from build123d import *

# Parameters (mm, degrees)
SKETCH1_R           = 7.9375
BOSS_EXTRUDE1_DEPTH = 42
SKETCH4_R           = 19
SKETCH4_R_2         = 2
BOSS_EXTRUDE3_DEPTH = 3.8
BOSS_EXTRUDE5_DEPTH = 19.8272
SKETCH7_R           = 7.9375
BOSS_EXTRUDE6_DEPTH = 24


with BuildPart() as part:
    # Sketch1 → Boss-Extrude1 (new body)
    with BuildSketch(Plane(origin=(0, 0, 0), x_dir=(0, 0, -1), z_dir=(1, 0, 0))):
        Circle(SKETCH1_R)
    extrude(amount=BOSS_EXTRUDE1_DEPTH)

    # Sketch4 → Boss-Extrude3 (add)
    with BuildSketch(Plane.ZY):
        Circle(SKETCH4_R)
        with Locations((-10.5, 10.5)):
            Circle(SKETCH4_R_2, mode=Mode.SUBTRACT)
        with Locations((10.5, 10.5)):
            Circle(SKETCH4_R_2, mode=Mode.SUBTRACT)
        with Locations((10.5, -10.5)):
            Circle(SKETCH4_R_2, mode=Mode.SUBTRACT)
        with Locations((-10.5, -10.5)):
            Circle(SKETCH4_R_2, mode=Mode.SUBTRACT)
    extrude(amount=BOSS_EXTRUDE3_DEPTH)

    # Sketch6 → Boss-Extrude5 (add)
    with BuildSketch(Plane(origin=(42, 0, 0), x_dir=(0, 0, -1), z_dir=(1, 0, 0))):
        with BuildLine():
            Line((-2.3815, 5.188813785), (2.3815, 5.188813785))
            Line((2.3815, 5.188813785), (2.3815, 7.571813785))
            ThreePointArc((2.3815, 7.571813785), (0, -7.9375), (-2.3815, 7.571813785))
            Line((-2.3815, 7.571813785), (-2.3815, 5.188813785))
        make_face()
    extrude(amount=BOSS_EXTRUDE5_DEPTH)

    # Sketch7 → Boss-Extrude6 (add)
    with BuildSketch(Plane(origin=(61.8272, 0, 0), x_dir=(0, 0, -1), z_dir=(1, 0, 0))):
        Circle(SKETCH7_R)
    extrude(amount=BOSS_EXTRUDE6_DEPTH)


solid = part.part
Part model, mm, in its own coordinate system. A direction names the side the tool comes from. Round coordinates to 2 decimals unless told otherwise and drop trailing zeros. Write each loop counter-clockwise with the first axis right and the second up, starting at its lowest first coordinate (ties: lowest second). Pieces come first, ordered by that corner, then holes. Notation, with made-up numbers: M 70.5,23 L 90.5,23 A20 cw 90.5,53 Z; hole C 50,56 d8. An arc over 180 degrees is marked long. Return JSON: item names as keys, results as strings. Group by question number.
(1) Pin check, flat tips, straight feed: pin 1 Ø0.7 at (x, y) = (49.5, 6.5) entering from +Z; pin 2 Ø6.5 at (y, z) = (-10.5, 10.5) entering from +X; pin 3 Ø1.2 at (x, y) = (51, 6) entering from -Z; pin 4 Ø3.5 at (y, z) = (10.5, -10.5) entering from +X. Stop position of each tip, or through.
(2) Saw through at B-B on y = 0. Write the cut outline in (x, z), then the cut area to 3 significant figures.
(3) Saw through at A-A on z = -10.5. Write the cut outline in (x, y).
(4) Two-plate mould, pull along X, no slides. Class faces 3 (the face through (0, 0.3, 8.2)), 4 (the face through (42, 7, 0)), 5 (the face through (-1.873, -9.148, 9.026)): +X half, -X half, draft (parallel to the pull), parting line (faces both ways), or undercut.
(5) Saw through at C-C on z = 0. Write the cut outline in (x, y).
(6) Which spindle directions (+Z, -Z, +X, -X, +Y, -Y) get a long thin tool onto all of the face, cutting with end or side? Do faces 1 (the face through (-1.873, -9.148, -11.974)), 2 (the face through (52, 6, 2.382)). Say none if no direction does.
(7) Drill centre lines: probe 1 along Z at (x, y) = (-1, -10); probe 2 along Y at (x, z) = (-2.4, 10.5); probe 3 along X at (y, z) = (-11, -5). Where is each one in solid material? Low to high.
Returned:
{
 "1": {"pin 1": "z = 5.02", "pin 2": "x = 0", "pin 3": "z = -5.82", "pin 4": "through"},
 "2": {"outline": "M -3.8,-19 L 0,-19 L 0,-7.94 L 85.83,-7.94 L 85.83,7.94 L 0,7.94 L 0,19 L -3.8,19 Z", "area": "1,510 mm²"},
 "3": {"outline": "M -3.8,-15.84 L 0,-15.84 L 0,-12.5 L -3.8,-12.5 Z; M -3.8,-8.5 L 0,-8.5 L 0,8.5 L -3.8,8.5 Z; M -3.8,12.5 L 0,12.5 L 0,15.84 L -3.8,15.84 Z"},
 "4": {"face 3": "+X half", "face 4": "undercut", "face 5": "draft"},
 "5": {"outline": "M -3.8,-19 L 0,-19 L 0,-7.94 L 85.83,-7.94 L 85.83,7.94 L 61.83,7.94 L 61.83,5.19 L 42,5.19 L 42,7.94 L 0,7.94 L 0,19 L -3.8,19 Z"},
 "6": {"face 1": "+X, -X", "face 2": "+Y"},
 "7": {"probe 1": "-16.16 to -12.44, -8.56 to 8.56, 12.44 to 16.16", "probe 2": "-15.84 to -12.5, -8.5 to 8.5, 12.5 to 15.84", "probe 3": "-3.8 to 0"}
}
